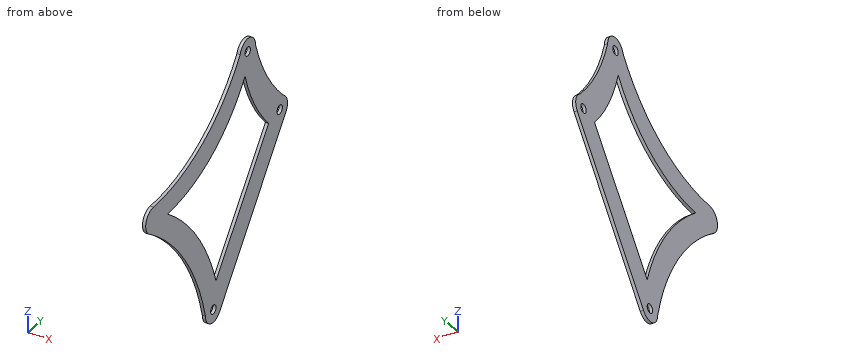
Autodesk Inventor part; units mm, degrees
ref_plane "YZ Plane" through (0, 0, 0) normal (1, 0, 0) x (0, 1, 0)
ref_plane "XZ Plane" through (0, 0, 0) normal (0, 1, 0) x (-1, 0, 0)
ref_plane "XY Plane" through (0, 0, 0) normal (0, 0, 1) x (1, 0, 0)
sketch "Sketch1" plane through (0, 0, 0) normal (1, 0, 0) x (0, 1, 0)
  circle A0 centre (-50.3348, 10.4318) radius 6.35
  circle A1 centre (25.9635, 53.6322) radius 2.1844
  circle A2 centre (51.8593, 11.1419) radius 2.1844
  circle A3 centre (-1.8993, -59.6622) radius 2.1844
  arc A4 (-31.4874, -97.6281) -> (-30.8803, -97.2439) centre (-31.376, -97.1325) ccw
  line L0 (-31.4874, -97.6281) -> (-35.0063, -96.8369)
  arc A5 (-29.1899, -99.915) -> (-29.797, -100.2992) centre (-29.3014, -100.4107) ccw
  arc A6 (-31.4874, -97.6281) -> (-30.8803, -97.2439) centre (-31.376, -97.1325) ccw
  line L1 (-35.0063, -96.8369) -> (-31.4874, -97.6281)
  arc A7 (-37.6774, -98.5273) -> (-38.0616, -97.9203) centre (-38.1731, -98.4159) ccw
  line L2 (-38.0616, -97.9203) -> (-39.8211, -97.5246)
  arc A8 (-29.1899, -99.915) -> (-29.797, -100.2992) centre (-29.3014, -100.4107) ccw
  arc A9 (-37.6774, -98.5273) -> (-38.0616, -97.9203) centre (-38.1731, -98.4159) ccw
  line L3 (-39.8211, -97.5246) -> (-38.0616, -97.9203)
  line L4 (-39.8211, -97.5246) -> (-38.0616, -97.9203)
  arc A10 (-29.1899, -99.915) -> (-29.797, -100.2992) centre (-29.3014, -100.4107) ccw
  arc A11 (-37.6774, -98.5273) -> (-38.0616, -97.9203) centre (-38.1731, -98.4159) ccw
  arc A12 (-29.1899, -99.915) -> (-29.797, -100.2992) centre (-29.3014, -100.4107) ccw
  arc A13 (-31.4874, -97.6281) -> (-30.8803, -97.2439) centre (-31.376, -97.1325) ccw
  line L5 (-31.4874, -97.6281) -> (-35.0063, -96.8369)
  arc A14 (-37.6774, -98.5273) -> (-38.0616, -97.9203) centre (-38.1731, -98.4159) ccw
  line L6 (-38.0616, -97.9203) -> (-39.8211, -97.5246)
  arc A15 (-31.4874, -97.6281) -> (-30.8803, -97.2439) centre (-31.376, -97.1325) ccw
  line L7 (-35.0063, -96.8369) -> (-31.4874, -97.6281)
  circle A16 centre (25.9635, 53.6322) radius 6.35
  circle A17 centre (51.8593, 11.1419) radius 6.35
  circle A18 centre (-1.8993, -59.6622) radius 6.35
  arc A19 (-50.3348, 16.7818) -> (19.8389, 55.3092) centre (-51.5807, 102.222) ccw
  arc A20 (32.3135, 53.6322) -> (54.7772, 16.7818) centre (116.2711, 79.5401) ccw
  arc A21 (-8.2493, -59.6622) -> (-53.2527, 4.7919) centre (-114.0974, -85.6296) ccw
  line L8 (3.2531, -63.3736) -> (56.9166, 7.3019)
  arc A22 (-38.9414, 7.3019) -> (23.7791, 42.5126) centre (-41.3896, 85.1299) ccw
  arc A23 (23.7791, 42.5126) -> (42.9324, 8.9575) centre (103.5332, 65.7926) ccw
  line L9 (42.9324, 8.9575) -> (0.2851, -46.536)
  arc A24 (0.2851, -46.536) -> (-38.9414, 7.3019) centre (-100.9359, -79.0766) ccw
  point P0 (0, 0)
  dimension "d0" = 12.7
  dimension "d1" = 12.7
  dimension "d2" = 12.7
  dimension "d3" = 12.7
extrude "Extrusion1" add sketch "Sketch1" along normal blind 1.5875
properties part number "ringblockerv2"
Can you work these out from the model? Positions are in its coordinate system, mm. Coordinates: 2 decimals unless noted, no trailing zeros. Write each loop counter-clockwise with the first axis right and the second up, starting at its lowest first coordinate (ties: lowest second). Pieces come first, ordered by that corner, then holes. Notation, with made-up numbers: (-35, 53.25) - (-11, 53.25) arc R30 ccw to (-11, 75.25) - close; hole circle Ø9 at (9.25, 54). An arc over 180 degrees is marked (long way). Return JSON: item names as keys, results as strings. Group by question number.
Item 1: If we section it at D-D (z = -52): Write out the boundary of the cut face in (x, y), then the cut area to 3 significant figures.
Item 2: If we section it at B-B (y = -10): Write out the boundary of the cut face in (x, z).
Item 3: I'm going to push a flat-ended pin straight in: pin 1 Ø3.5 at (y, z) = (-1.9, -59.66) entering from +X. Where does the tip first touch, or does it pass through?
Item 4: If we section it at C-C (x = 1.3): Write out the boundary of the cut face in (y, z), then the cut area to 3 significant figures.
Item 5: Please list where these lines run through material, in increasing order: probe 1 along Z at (x, y) = (0.55, 4); probe 2 along Y at (x, z) = (0.65, 1.5); probe 3 along Y at (x, z) = (0.85, -61).
Item 6: If we section it at A-A (z = -1.5): Write out the boundary of the cut face in (x, y).
Return value:
{
 "1": {"outline": "(0, -10.43) - (1.59, -10.43) - (1.59, 11.89) - (0, 11.89) - close", "area": "35.4 mm^2"},
 "2": {"outline": "(0, -53.35) - (1.59, -53.35) - (1.59, -23.98) - (0, -23.98) - close; (0, 13.87) - (1.59, 13.87) - (1.59, 27.57) - (0, 27.57) - close"},
 "3": {"pin 1": "passes through"},
 "4": {"outline": "(-53.25, 4.79) arc R108.99 cw to (-8.25, -59.66) arc R6.35 ccw to (3.25, -63.37) - (56.92, 7.3) arc R6.35 ccw to (54.78, 16.78) arc R87.86 cw to (32.31, 53.63) arc R6.35 ccw to (19.84, 55.31) arc R85.45 cw to (-50.33, 16.78) arc R6.35 ccw to start; hole (-38.94, 7.3) arc R106.32 cw to (0.29, -46.54) - (42.93, 8.96) arc R83.08 cw to (23.78, 42.51) arc R77.87 cw to start; hole circle Ø4.37 at (-1.9, -59.66); hole circle Ø4.37 at (25.96, 53.63); hole circle Ø4.37 at (51.86, 11.14)", "area": "3,710 mm^2"},
 "5": {"probe 1": "z = -62.39 to -41.7, 21.86 to 37.32", "probe 2": "y = -48.63 to -31.57, 37.2 to 52.51", "probe 3": "y = -8.11 to -3.63, -0.17 to 5.06"},
 "6": {"outline": "(0, -44.81) - (1.59, -44.81) - (1.59, -28.23) - (0, -28.23) - close; (0, 34.9) - (1.59, 34.9) - (1.59, 50.23) - (0, 50.23) - close"}
}
